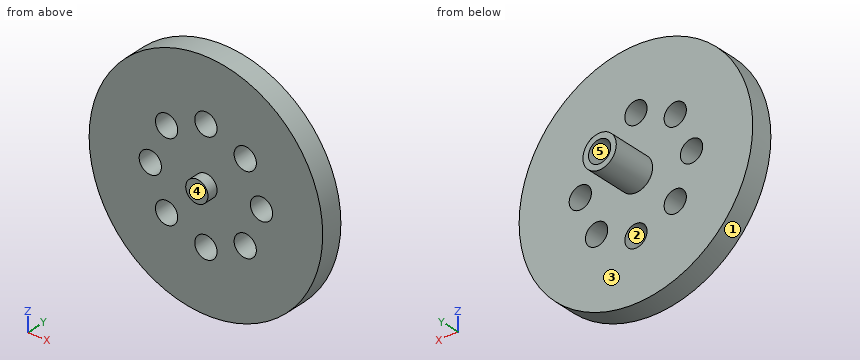
from build123d import *

# Parameters (mm, degrees)
F0_R     = 16.66875
F1_DEPTH = 3.175
F2_R     = 2.38125
F3_DEPTH = 6.35
F4_R     = 1.5875
F5_DEPTH = 25.4
F6_R     = 1.5875
F7_DEPTH = 1.5875
F8_R     = 1.5875
F9_DEPTH = 3.81


with BuildPart() as f1:
    # F0 (on Front) → F1 (new body)
    with BuildSketch(Plane.XZ):
        Circle(F0_R)
    extrude(amount=-F1_DEPTH)

    # F2 (on face) → F3 (join)
    with BuildSketch(Plane(origin=(0, 3.175, 0), x_dir=(-1, 0, 0), z_dir=(0, 1, 0))):
        Circle(F2_R)
    extrude(amount=F3_DEPTH)

    # F4 (on face) → F5 (cut)
    with BuildSketch(Plane(origin=(0, 9.525, 0), x_dir=(-1, 0, 0), z_dir=(0, 1, 0))):
        with Locations((7.9375, 0)):
            Circle(F4_R)
        with Locations((5.61266, 5.61266)):
            Circle(F4_R)
        with Locations((0, 7.9375)):
            Circle(F4_R)
        with Locations((-5.61266, 5.61266)):
            Circle(F4_R)
        with Locations((-7.9375, 0)):
            Circle(F4_R)
        with Locations((-5.61266, -5.61266)):
            Circle(F4_R)
        with Locations((0, -7.9375)):
            Circle(F4_R)
        with Locations((5.61266, -5.61266)):
            Circle(F4_R)
    extrude(amount=-F5_DEPTH, mode=Mode.SUBTRACT)

    # F6 (on face) → F7 (join)
    with BuildSketch(Plane.XZ):
        Circle(F6_R)
    extrude(amount=F7_DEPTH)

    # F8 (on face) → F9 (cut)
    with BuildSketch(Plane(origin=(0, 9.525, 0), x_dir=(-1, 0, 0), z_dir=(0, 1, 0))):
        Circle(F8_R)
    extrude(amount=-F9_DEPTH, mode=Mode.SUBTRACT)


solid = f1.part
For this review, take the finished solid that the model builds, in its own axes (mm). Face numbers are marked on the shaded views. A direction names the side the tool comes from. Round coordinates to 2 decimals unless told otherwise and drop trailing zeros. Write each loop counter-clockwise with the first axis right and the second up, starting at its lowest first coordinate (ties: lowest second). Pieces come first, ordered by that corner, then holes. Notation, with made-up numbers: (59, 38.5) -> (74, 38.5) arc R17 cw to (74, 56.5) -> close; hole circle Ø11 at (70.25, 77). An arc over 180 degrees is marked (long way). Use CSV: the item, a comma, the result in double quotes.
(1) Draft analysis for pull direction Z (two halves, no side actions). For the marked faces 1, 2 and 3, state which applies: +Z half, -Z half, draft (parallel to the pull), parting line (faces both ways), or undercut.
Computed values:
face 1,"parting line"
face 2,"undercut"
face 3,"draft"
(2) To check wall thickness, follow L1, parallel to Z at x = 0, y = 1.15 (3 decimals); L2, parallel to X at y = 3, z = 5; L3, parallel to Z at x = 0, y = 7.95. State the ranges of each line that lie inside material, in increasing order. Write a range as [from, to].
Computed values:
L1,"[-16.669, -9.525], [-6.35, 6.35], [9.525, 16.669]"
L2,"[-15.9, -7.08], [-4.15, 4.15], [7.08, 15.9]"
L3,"[-2.38, -1.59], [1.59, 2.38]"
(3) For the marked faces 4 and 5, list the 3-axis set-ups (+Z, -Z, +X, -X, +Y, -Y) from which the entire face can be reached by the end or side of a thin tool; tool diameter is ignored.
Computed values:
face 4,"+Z, -Z, +X, -X, -Y"
face 5,"+Y"
(4) Clearance check with flat-ended pins moving along their axes: P1, Ø4, axis at x = 5.61, z = -5.61, coming from the +Y side (3 decimals); P2, Ø5, axis at x = -5.61, z = -5.61, coming from the -Y side; P3, Ø6, axis at y = 2, z = -13, coming from the +X side. State where each tip first meets the part, or that it passes through.
Computed values:
P1,"y = 3.175"
P2,"y = 0"
P3,"x = 13.34"
(5) Consider section D-D, the plane y = 4.5. Give the boundary of the cut face in (x, z), plus the area to 3 significant figures.
Computed values:
outline,"circle Ø4.76 at (0, 0)"
area,"17.8 mm²"
(6) Consider section C-C, the plane z = 9. Give the boundary of the cut face in (x, y) (3 decimals).
Computed values:
outline,"(-14.03, 0) -> (-1.18, 0) -> (-1.18, 3.175) -> (-14.03, 3.175) -> close; (1.18, 0) -> (14.03, 0) -> (14.03, 3.175) -> (1.18, 3.175) -> close"
(7) Consider section A-A, the plane z = 0. Give the number of separate pieces and of enclosed holes in the cut face, plus the area to 3 significant figures.
Computed values:
separate pieces,"3"
enclosed holes,"0"
area,"109 mm²"
